Geometry check sheet. Reference: the model listing, model coordinates, mm. Round coordinates to 2 decimals unless told otherwise and drop trailing zeros. Order: outer loops, then holes, each group sorted by start corner. A loop starts at its lowest first (then second) coordinate and runs counter-clockwise, first axis right, second up.
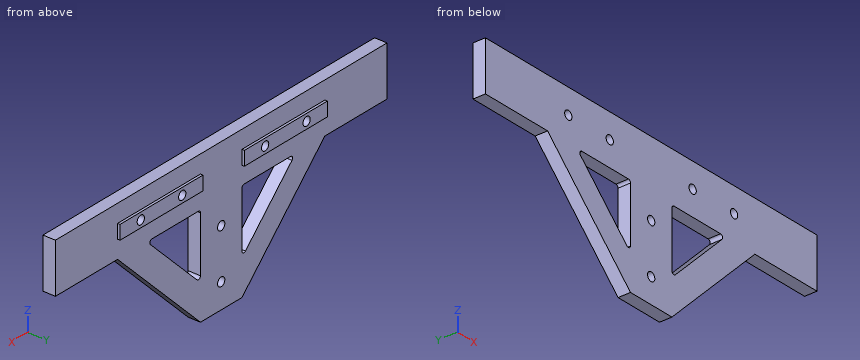
```python
from build123d import *

# Parameters (mm, degrees)
ESBO_O1_R                = 1.75
RESSALTO_EXTRUS_O1_DEPTH = 5
ESBO_O3_W                = 40
ESBO_O3_H                = 5.65
ESBO_O3_R                = 1.75
RESSALTO_EXTRUS_O2_DEPTH = 1
ESBO_O4_W                = 30
ESBO_O4_H                = 20.000002677
RESSALTO_EXTRUS_O3_DEPTH = 5


with BuildPart() as part:
    # Esboço1 → Ressalto-extrusão1 (new body)
    with BuildSketch(Plane(origin=(0, 0, 0), x_dir=(1, 0, 0), z_dir=(0, 1, 0))):
        Polygon((-50, 0), (-50, 20.000002677), (-9.999996661, 60.000002546), (9.999996661, 60.000002546), (50, 20.000002677), (50, 0), align=None)
        with Locations(Location((-40, 10.000001339, 0), (0, 0, 270))):
            Circle(ESBO_O1_R, mode=Mode.SUBTRACT)
        with Locations(Location((-20, 10.000001339, 0), (0, 0, 270))):
            Circle(ESBO_O1_R, mode=Mode.SUBTRACT)
        with Locations(Location((0, 50.000002546, 0), (0, 0, 270))):
            Circle(ESBO_O1_R, mode=Mode.SUBTRACT)
        with Locations(Location((0, 30.000002546, 0), (0, 0, 270))):
            Circle(ESBO_O1_R, mode=Mode.SUBTRACT)
        with Locations(Location((20, 10.000001339, 0), (0, 0, 90))):
            Circle(ESBO_O1_R, mode=Mode.SUBTRACT)
        with Locations(Location((40, 10.000001339, 0), (0, 0, 90))):
            Circle(ESBO_O1_R, mode=Mode.SUBTRACT)
        with BuildLine():
            Line((-10, 43.443650782), (-10, 21.000001339))
            ThreePointArc((-10, 21.000001339), (-10.292893219, 20.292894558), (-11, 20.000001339))
            Line((-11, 20.000001339), (-33.443651391, 20.000001339))
            ThreePointArc((-33.443651391, 20.000001339), (-34.367530932, 20.617317926), (-34.150758141, 21.707108151))
            Line((-34.150758141, 21.707108151), (-11.707106751, 44.150757594))
            ThreePointArc((-11.707106751, 44.150757594), (-10.617316548, 44.367530307), (-10, 43.443650782))
        make_face(mode=Mode.SUBTRACT)
        with BuildLine():
            Line((11.707106751, 44.150757594), (34.150758141, 21.707108151))
            ThreePointArc((34.150758141, 21.707108151), (34.367530932, 20.617317926), (33.443651391, 20.000001339))
            Line((33.443651391, 20.000001339), (11, 20.000001339))
            ThreePointArc((11, 20.000001339), (10.292893219, 20.292894558), (10, 21.000001339))
            Line((10, 21.000001339), (10, 43.443650782))
            ThreePointArc((10, 43.443650782), (10.617316548, 44.367530307), (11.707106751, 44.150757594))
        make_face(mode=Mode.SUBTRACT)
    extrude(amount=RESSALTO_EXTRUS_O1_DEPTH)

    # Esboço3 → Ressalto-extrusão2 (add)
    # profile 1 of 2: a face of its own
    with BuildSketch(Plane(origin=(0, 5, 0), x_dir=(1, 0, 0), z_dir=(0, 1, 0))):
        with Locations((-30, 10.000001339)):
            Rectangle(ESBO_O3_W, ESBO_O3_H)
        with Locations(Location((-40, 10.000001339, 0), (0, 0, 270))):
            Circle(ESBO_O3_R, mode=Mode.SUBTRACT)
        with Locations(Location((-20, 10.000001339, 0), (0, 0, 270))):
            Circle(ESBO_O3_R, mode=Mode.SUBTRACT)
    # profile 2 of 2: a face of its own
    with BuildSketch(Plane(origin=(0, 5, 0), x_dir=(1, 0, 0), z_dir=(0, 1, 0))):
        with Locations((30, 10.000001339)):
            Rectangle(ESBO_O3_W, ESBO_O3_H)
        with Locations(Location((20, 10.000001339, 0), (0, 0, 90))):
            Circle(ESBO_O3_R, mode=Mode.SUBTRACT)
        with Locations(Location((40, 10.000001339, 0), (0, 0, 90))):
            Circle(ESBO_O3_R, mode=Mode.SUBTRACT)
    extrude(amount=RESSALTO_EXTRUS_O2_DEPTH)

    # Esboço4 → Ressalto-extrusão3 (add)
    with BuildSketch(Plane.XZ):
        with Locations((-65, -10.000001339)):
            Rectangle(ESBO_O4_W, ESBO_O4_H)
        with Locations((65, -10.000001339)):
            Rectangle(ESBO_O4_W, ESBO_O4_H)
    extrude(amount=-RESSALTO_EXTRUS_O3_DEPTH)


solid = part.part
```
(1) Sectioned sample at A-A, the plane x = 40. Record the cut outline in (y, z) (3 decimals).
Returned:
outline: (0, -30) - (5, -30) - (5, -12.825) - (6, -12.825) - (6, -11.75) - (0, -11.75) - close; (0, -8.25) - (6, -8.25) - (6, -7.175) - (5, -7.175) - (5, 0) - (0, 0) - close
(2) Material ranges on line 1 (X direction, y = 4, z = -40.5); line 2 (X direction, y = 4.55, z = -34.5); line 3 (Z direction, x = 20, y = 1.3), recorded low to high.
Returned:
line 1: x = -29.5 to -15.36, -10 to 10, 15.36 to 29.5
line 2: x = -35.5 to -21.36, -10 to 10, 21.36 to 35.5
line 3: z = -50 to -35.86, -20 to -11.75, -8.25 to 0
(3) Sectioned sample at C-C, the plane x = 0. Record the cut outline in (y, z).
Returned:
outline: (0, -60) - (5, -60) - (5, -51.75) - (0, -51.75) - close; (0, -48.25) - (5, -48.25) - (5, -31.75) - (0, -31.75) - close; (0, -28.25) - (5, -28.25) - (5, 0) - (0, 0) - close
(4) Depth check by flat-ended pin: P1, Ø3, axis at x = -40, z = -10, coming from the -Y side; P2, Ø0.8, axis at x = -23, y = 5.5, coming from the -Z side (3 decimals); P3, Ø2, axis at y = 1.5, z = -28, coming from the +X side; P4, Ø2, axis at y = 3, z = -39, coming from the -X side. Enter the tip coordinate at first touch or a pass-through.
Returned:
P1: passes through
P2: stops at z = -12.825
P3: stops at x = 43
P4: stops at x = -32
(5) Sectioned sample at B-B, the plane y = 3.95. Give the number of separate pieces and of enclosed holes in the cut face, and give its area (3 significant figures).
Returned:
separate pieces: 1
enclosed holes: 8
area: 4,880 mm2
(6) Sectioned sample at D-D, the plane z = -26. Record the cut outline in (x, y).
Returned:
outline: (-44, 0) - (-29.86, 0) - (-29.86, 5) - (-44, 5) - close; (-10, 0) - (10, 0) - (10, 5) - (-10, 5) - close; (29.86, 0) - (44, 0) - (44, 5) - (29.86, 5) - close
